from build123d import *

# Parameters (mm, degrees)
F1_W     = 30.5479690433
F1_H     = 33.1509709358
F1_W_2   = 16.4528656751
F1_H_2   = 12.8562636673
F1_R     = 3.862880512
F2_DEPTH = 12.7


with BuildPart() as f2:
    # F1 (on face) → F2 (new body)
    with BuildSketch(Plane.XY):
        Rectangle(F1_W, F1_H)
        Rectangle(F1_W_2, F1_H_2, mode=Mode.SUBTRACT)
        Rectangle(F1_W_2, F1_H_2)
        Circle(F1_R, mode=Mode.SUBTRACT)
    extrude(amount=F2_DEPTH)


solid = f2.part
For this review, take the finished solid that the model builds, in its own axes (mm). Round coordinates to 2 decimals unless told otherwise and drop trailing zeros. Write each loop counter-clockwise with the first axis right and the second up, starting at its lowest first coordinate (ties: lowest second). Pieces come first, ordered by that corner, then holes. Notation, with made-up numbers: (36.5, 80.25) -> (78.5, 80.25) arc R22 cw to (78.5, 108.25) -> close; hole circle Ø4 at (-35, 0). An arc over 180 degrees is marked (long way). Put each result on its own line as item: value.
Q1. Consider section C-C on z = 3.5. State the section outline as (x, y) points.
Determined:
outline: (-15.27, -16.58) -> (15.27, -16.58) -> (15.27, 16.58) -> (-15.27, 16.58) -> close; hole circle Ø7.73 at (0, 0)
Q2. Consider section A-A on y = 0. State the section outline as (x, z) points, and give its area (3 significant figures).
Determined:
outline: (-15.27, 0) -> (-3.86, 0) -> (-3.86, 12.7) -> (-15.27, 12.7) -> close; (3.86, 0) -> (15.27, 0) -> (15.27, 12.7) -> (3.86, 12.7) -> close
area: 290 mm^2
Q3. Consider section B-B on x = 0. State the section outline as (y, z) points, and give its area (3 significant figures).
Determined:
outline: (-16.58, 0) -> (-3.86, 0) -> (-3.86, 12.7) -> (-16.58, 12.7) -> close; (3.86, 0) -> (16.58, 0) -> (16.58, 12.7) -> (3.86, 12.7) -> close
area: 323 mm^2
Q4. To check wall thickness, follow L1, parallel to Y at x = 0, z = 5.25; L2, parallel to X at y = 1.5, z = 2.25; L3, parallel to X at y = 0.5, z = 12. State the ranges of each line that lie inside material, in increasing order. Write a range as [from, to].
Determined:
L1: y = [-16.58, -3.86], [3.86, 16.58]
L2: x = [-15.27, -3.56], [3.56, 15.27]
L3: x = [-15.27, -3.83], [3.83, 15.27]
